For this review, take the finished solid that the model builds, in its own axes (mm). A direction names the side the tool comes from. Give positions to 0.01 mm unless a question says otherwise; leave off trailing zeros. Order: outer loops, then holes, each group sorted by start corner. A loop starts at its lowest first (then second) coordinate and runs counter-clockwise, first axis right, second up. Notation, with made-up numbers: (9.25, -24) - (14.25, -24) arc R21 ccw to (14.25, 10) - close; hole circle Ø11 at (29.25, 28). An arc over 180 degrees is marked (long way). Put each result on its own line as item: value. Start each with the question number.
```python
from build123d import *

# Parameters (mm, degrees)
F0_W     = 46.9391979277
F0_H     = 111.8616014719
F3_DEPTH = 25.4
F4_DEPTH = 25.4
F5_DEPTH = 25.4
F6_SIZE  = 5.08


with BuildPart() as f3:
    # F0 (on Front) → F3 (new body)
    with BuildSketch(Plane.XZ):
        Rectangle(F0_W, F0_H)
    extrude(amount=F3_DEPTH)

    # F1 (on face) → F4 (join)
    with BuildSketch(Plane.XZ):
        Polygon((-54.4846235865, 32.6140428748), (0, 0), (54.4846235865, 32.6140428748), (0, 65.2280857495), align=None)
    extrude(amount=F4_DEPTH)

    # F2 (on Front) → F5 (join)
    with BuildSketch(Plane.XZ):
        Polygon((-40.705913781, -30.3919164129), (0, -60.7838328259), (40.705913781, -30.3919164129), (0, 0), align=None)
    extrude(amount=F5_DEPTH)

    # F6
    f6_edges = [f3.edges().sort_by_distance(p)[0] for p in [
        (-38.977111, -25.4, 23.331375),
        (-23.469599, -25.4, -1.737102),
        (-32.087756, -25.4, -23.957414),
        (-32.087756, -25.4, -36.826419),
        (-23.469599, -25.4, -49.595861),
        (-14.984794, -25.4, -55.930801),
        (-3.249994, -25.4, -58.357317),
        (14.984794, -25.4, -55.930801),
        (23.469599, -25.4, -49.595861),
        (32.087756, -25.4, -36.826419),
        (32.087756, -25.4, -23.957414),
        (23.469599, -25.4, -1.737102),
        (38.977111, -25.4, 23.331375),
        (38.977111, -25.4, 41.896711),
        (23.469599, -25.4, 53.55509),
        (19.500765, -25.4, 55.930801),
        (7.765966, -25.4, 60.579443),
        (-7.765966, -25.4, 60.579443),
        (-19.500765, -25.4, 55.930801),
        (-23.469599, -25.4, 53.55509),
        (-38.977111, -25.4, 41.896711),
    ]]
    chamfer(f6_edges, length=F6_SIZE)


solid = f3.part
```
1. Tool access review of faces 1 (the face through (-31.97, -10.02, -23.87)), 2 (the face through (19, -10, 55.931)), 3 (the face through (23.47, -10, -50)), 4 (the face through (38.76, -10.02, 23.2)), 5 (the face through (36.221, -22.824, 24.6)): name each direction out of +Z, -Z, +X, -X, +Y, -Y from which nothing blocks a thin tool from reaching the whole face with its end or side.
2. Add section C-C, the plane y = -11.25. Give the boundary of the cut face in (x, z), then the cut area to 3 significant figures.
3. Clearance check with flat-ended pins moving along their axes: pin 1 (2.5 mm diameter, centred on y = -12, z = 54, fed in from +X); pin 2 (8.5 mm diameter, centred on x = 12.5, y = -11, fed in from -Z); pin 3 (6.5 mm diameter, centred on x = -21, y = -6.5, fed in from +Z); pin 4 (1.5 mm diameter, centred on x = 1, z = -30, fed in from +Y). State where each tip first meets the part, or that it passes through.
4. Wall thickness on line 1 (Z direction, x = 21, y = -19.75); line 2 (Z direction, x = -27, y = -10.25); line 3 (X direction, y = -19, z = -52): over which ranges is each line inside the solid? List them lowest first. Write a range as from..to.
5. Add section D-D, the plane x = -12. Give the boundary of the cut face in (y, z), then the cut area to 3 significant figures.
6. Add section A-A, the plane x = -27.5. Give the boundary of the cut face in (y, z), then the cut area to 3 significant figures.
7. Add section B-B, the plane z = -1. Give the boundary of the cut face in (x, y), then the cut area to 3 significant figures.
Found:
1. face 1: -X, +Y, -Y
1. face 2: +Z, +X, +Y, -Y
1. face 3: -Z, +X, +Y, -Y
1. face 4: +X, +Y, -Y
1. face 5: +X, -Y
2. outline: (-54.48, 32.61) - (-23.47, 14.05) - (-23.47, -17.52) - (-40.71, -30.39) - (-23.47, -43.26) - (-23.47, -55.93) - (-6.5, -55.93) - (0, -60.78) - (6.5, -55.93) - (23.47, -55.93) - (23.47, -43.26) - (40.71, -30.39) - (23.47, -17.52) - (23.47, 14.05) - (54.48, 32.61) - (23.47, 51.18) - (23.47, 55.93) - (15.53, 55.93) - (0, 65.23) - (-15.53, 55.93) - (-23.47, 55.93) - (-23.47, 51.18) - close
2. area: 7,020 mm^2
3. pin 1: stops at x = 23.47
3. pin 2: stops at z = -55.93
3. pin 3: stops at z = 55.93
3. pin 4: stops at y = 0
4. line 1: z = -55.93..55.93
4. line 2: z = -40.63..-20.16, 16.16..49.07
4. line 3: x = -23.47..23.47
5. outline: (-25.4, -50.85) - (-20.32, -55.93) - (0, -55.93) - (0, 58.04) - (-20.32, 58.04) - (-25.4, 52.12) - close
5. area: 2,870 mm^2
6. outline: (-25.4, -33.91) - (-20.32, -40.25) - (0, -40.25) - (0, -20.53) - (-20.32, -20.53) - (-25.4, -26.87) - close; (-25.4, 22.38) - (-20.32, 16.46) - (0, 16.46) - (0, 48.77) - (-20.32, 48.77) - (-25.4, 42.85) - close
6. area: 1,260 mm^2
7. outline: (-23.47, -20.32) - (-18.39, -25.4) - (18.39, -25.4) - (23.47, -20.32) - (23.47, 0) - (-23.47, 0) - close
7. area: 1,170 mm^2
